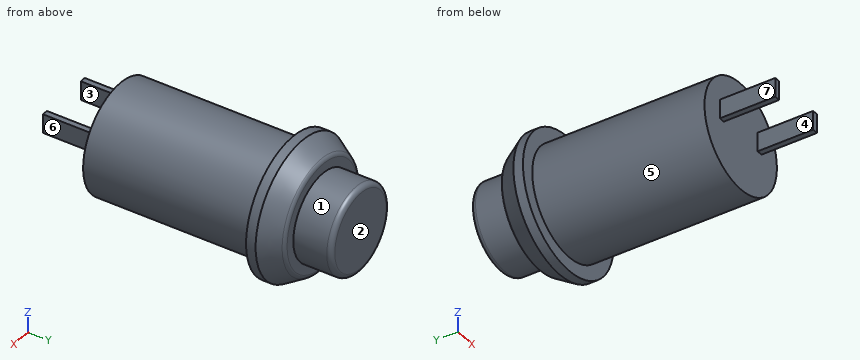
from build123d import *

# Parameters (mm, degrees)
FILLET1_R           = 0.5
SKETCH2_W           = 0.6
SKETCH2_H           = 2
BOSS_EXTRUDE1_DEPTH = 5.8


with BuildPart() as part:
    # Sketch1 → Revolve1 (revolve)
    with BuildSketch(Plane.XY, mode=Mode.PRIVATE) as revolve1_sk:
        Polygon((0, 0), (-5.65, 0), (-5.65, 18), (-7.1, 18), (-7.1, 19), (-5.75, 21.2), (-4.5, 21.2), (-4.5, 25.2), (0, 25.2), align=None)
    revolve(revolve1_sk.sketch.rotate(Axis((0, 0, 0), (0, 1, 0)), 270), axis=Axis((0, 0, 0), (0, 1, 0)))

    # Fillet1
    fillet1_edges = [part.edges().sort_by_distance(p)[0] for p in [
        (0, 25.2, 4.5),
        (0, 21.2, 5.75),
    ]]
    fillet(fillet1_edges, radius=FILLET1_R)

    # Sketch2 → Boss-Extrude1 (add)
    with BuildSketch(Plane.XZ):
        with Locations((-2.95, 1)):
            Rectangle(SKETCH2_W, SKETCH2_H)
        with Locations((2.95, 1)):
            Rectangle(SKETCH2_W, SKETCH2_H)
    extrude(amount=BOSS_EXTRUDE1_DEPTH)


solid = part.part
Check sheet for the modelled part. Datum: model origin and axes. Units: mm. Face numbers are marked on the shaded views. A direction names the side the tool comes from. Give positions to 0.01 mm unless a question says otherwise; leave off trailing zeros. Loops run counter-clockwise (first coordinate to the right, second up) from the corner with the lowest first, then second, coordinate; pieces in that order, holes last. Notation, with made-up numbers: M 34.25,14 L 92.25,14 A19 cw 92.25,29 Z; hole C 22.5,-18 d5. An arc over 180 degrees is marked long. Return JSON: item names as keys, results as strings. Group by question number.
1. Thickness scan on L1, parallel to Y at x = 4.75, z = 0.75; L2, parallel to Y at x = 1, z = -2; L3, parallel to X at y = 10, z = -0.25. Record the ranges inside material, lowest first.
2. Cross-section at C-C on y = 11. Record the boundary of the cut face in (x, z), plus the area to 3 significant figures.
3. Cross-section at A-A on y = -1. Record the boundary of the cut face in (x, z), plus the area to 3 significant figures.
4. Cross-section at B-B on x = 0. Record the boundary of the cut face in (y, z).
5. Tool access check on the marked faces 4, 5, 6 and 7. Record the directions out of +Z, -Z, +X, -X, +Y, -Y that give a thin tool (end or side, any length) a straight path to the whole face; none if there is none.
6. Go/stop test with flat-tipped pins: pin 1 (1 mm diameter, centred on y = -4, z = 1, fed in from +X); pin 2 (0.5 mm diameter, centred on x = 3, y = -3, fed in from +Z); pin 3 (2 mm diameter, centred on x = 0, y = 10.5, fed in from -Z). Record where each tip stops, or that it passes through.
7. Mould release check, pull along X, two halves, no side actions. Record for the marked faces 1, 2 and 3: released by +X, released by -X, zero draft, split by the parting line, or undercut.
Return value:
{
 "1": {"L1": "0 to 21.2", "L2": "0 to 25.2", "L3": "-5.64 to 5.64"},
 "2": {"outline": "C 0,0 d11.3", "area": "100 mm^2"},
 "3": {"outline": "M -3.25,0 L -2.65,0 L -2.65,2 L -3.25,2 Z; M 2.65,0 L 3.25,0 L 3.25,2 L 2.65,2 Z", "area": "2.40 mm^2"},
 "4": {"outline": "M 0,-5.65 L 18,-5.65 L 18,-7.1 L 19,-7.1 L 20.96,-5.9 A0.5 ccw 21.2,-5.47 L 21.2,-4.5 L 24.7,-4.5 A0.5 ccw 25.2,-4 L 25.2,4 A0.5 ccw 24.7,4.5 L 21.2,4.5 L 21.2,5.47 A0.5 ccw 20.96,5.9 L 19,7.1 L 18,7.1 L 18,5.65 L 0,5.65 Z"},
 "5": {"face 4": "+Z, -Z, -Y", "face 5": "-Y", "face 6": "+Z, -Z, +X, -Y", "face 7": "+Z, -Z, -X, -Y"},
 "6": {"pin 1": "x = 3.25", "pin 2": "z = 2", "pin 3": "z = -5.65"},
 "7": {"face 1": "split by the parting line", "face 2": "zero draft", "face 3": "undercut"}
}
